from build123d import *

# Parameters (mm, degrees)
F0_W      = 36
F0_H      = 100
F1_DEPTH  = 89
F2_R      = 10.25
F3_DEPTH  = 25
F4_R      = 35.25
F5_DEPTH  = 27.5
F6_R      = 15.75
F7_DEPTH  = 3.5
F8_W      = 31.5
F8_H      = 105
F9_DEPTH  = 3.5
F10_R     = 8
F11_DEPTH = 8
F13_D     = 6.7564
F13_DEPTH = 26
F13_TIP   = 2.0298273432
F15_D     = 6.7564
F15_DEPTH = 26
F15_TIP   = 2.0298273432


with BuildPart() as f1:
    # F0 (on Top) → F1 (new body)
    with BuildSketch(Plane.XY):
        Rectangle(F0_W, F0_H)
    extrude(amount=F1_DEPTH)

    # F2 (on Front) → F3 (cut, symmetric)
    with BuildSketch(Plane.XZ):
        Circle(F2_R)
    extrude(amount=F3_DEPTH, both=True, mode=Mode.SUBTRACT)

    # F4 (on Right) → F5 (cut, symmetric)
    with BuildSketch(Plane.YZ):
        Circle(F4_R)
    extrude(amount=F5_DEPTH, both=True, mode=Mode.SUBTRACT)

    # F6 (on face) → F7 (join)
    with BuildSketch(Plane.XY.offset(89)):
        with Locations((0, 52.5)):
            Circle(F6_R)
        with Locations((0, -52.5)):
            Circle(F6_R)
    extrude(amount=-F7_DEPTH)

    # F8 (on face) → F9 (join)
    with BuildSketch(Plane.XY.offset(89)):
        Rectangle(F8_W, F8_H)
    extrude(amount=-F9_DEPTH)

    # F10 (on face) → F11 (join)
    with BuildSketch(Plane.XY.offset(89)):
        with Locations((0, 51.5)):
            Circle(F10_R)
        with Locations((0, -51.5)):
            Circle(F10_R)
    extrude(amount=-F11_DEPTH)

    # F13
    with Locations(Plane(origin=(0, 0, 0), x_dir=(1, 0, 0), z_dir=(0, 0, -1))):
        with Locations((0, 42.625)):
            Hole(F13_D / 2, depth=F13_DEPTH)
            with Locations((0, 0, -(F13_DEPTH + F13_TIP / 2))):  # 118° drill point
                Cone(0, F13_D / 2, F13_TIP, mode=Mode.SUBTRACT)

    # F15
    with Locations(Plane(origin=(0, 0, 0), x_dir=(1, 0, 0), z_dir=(0, 0, -1))):
        with Locations((0, -42.625)):
            Hole(F15_D / 2, depth=F15_DEPTH)
            with Locations((0, 0, -(F15_DEPTH + F15_TIP / 2))):  # 118° drill point
                Cone(0, F15_D / 2, F15_TIP, mode=Mode.SUBTRACT)


solid = f1.part
Can you work these out from the model? Positions are in its coordinate system, mm. A direction names the side the tool comes from. Round coordinates to 2 decimals unless told otherwise and drop trailing zeros. Loops run counter-clockwise (first coordinate to the right, second up) from the corner with the lowest first, then second, coordinate; pieces in that order, holes last. Notation, with made-up numbers: (37.25, 78.25) - (83.25, 78.25) arc R29 ccw to (83.25, 103.25) - close; hole circle Ø11 at (65.25, 27.25). An arc over 180 degrees is marked (long way). Use CSV: the item, a comma, the result in double quotes. Start each with the question number.
1) For faces 4 (the flat face through (0, 54, 81)), 5 (the flat face through (0, 61, 85.5)), 6 (the cylindrical face through (-1.6, 45.6, 13.2)), which set-ups out of +Z, -Z, +X, -X, +Y, -Y let a thin tool reach every point of the face, with its end or its side?
2) For pin 1 Ø5 at (x, y) = (1, 54) entering from -Z; pin 2 Ø1.2 at (y, z) = (51.5, 88) entering from +X; pin 3 Ø5.5 at (x, y) = (0, -42.625) entering from -Z, each with a flat end and sliding along its axis, tell me the tip position at first contact or that it passes through.
3) If we section it at D-D on x = -6: Write out the boundary of the cut face in (y, z).
4) We'd pull the mould along Y, two halves only. Please class faces 1 (the cylindrical face through (-0.346, -68.246, 87.274)), 2 (the conical face through (-0.127, -42.052, 27.677)), 3 (the flat face through (0, -39, 0)): released by +Y, released by -Y, zero draft, split by the parting line, or undercut.
5) Please list where these lines run through material, in increasing order: probe 1 along Y at (x, z) = (0, 5.5); probe 2 along Y at (x, z) = (0, 18); probe 3 along Z at (x, y) = (11, -56.5). Write a range as [from, to].
6) If we section it at B-B on y = 0: Write out the boundary of the cut face in (x, z).
7) If we section it at C-C on z = 83.5: Write out the boundary of the cut face in (x, y), plus the area to 3 significant figures.
8) If we section it at A-A on z = 22: Write out the boundary of the cut face in (x, y) (3 decimals), plus the area to 3 significant figures.
Geometry results:
1,face 4,"-Z, +X, -X, +Y"
1,face 5,"-Z, +Y"
1,face 6,"-Z"
2,pin 1,"stops at z = 81"
2,pin 2,"stops at x = 15.75"
2,pin 3,"stops at z = 26.38"
3,outline,"(-67.06, 85.5) - (-56.79, 85.5) - (-56.79, 81) - (-50, 81) - (-50, 0) - (-35.25, 0) arc R35.25 cw to (35.25, 0) - (50, 0) - (50, 81) - (56.79, 81) - (56.79, 85.5) - (67.06, 85.5) - (67.06, 89) - (-67.06, 89) - close"
4,face 1,"released by -Y"
4,face 2,"undercut"
4,face 3,"zero draft"
5,probe 1,"y = [-50, -46], [-39.25, -34.82], [34.82, 39.25], [46, 50]"
5,probe 2,"y = [-50, -46], [-39.25, -30.31], [30.31, 39.25], [46, 50]"
5,probe 3,"z = [85.5, 89]"
6,outline,"(-18, 35.25) - (18, 35.25) - (18, 89) - (-18, 89) - close"
7,outline,"(-18, -50) - (-7.86, -50) arc R8 ccw (long way) to (7.86, -50) - (18, -50) - (18, 50) - (7.86, 50) arc R8 ccw (long way) to (-7.86, 50) - (-18, 50) - close"
7,area,"3,850 mm2"
8,outline,"(-18, -50) - (18, -50) - (18, -27.542) - (-18, -27.542) - close; (-18, 27.542) - (18, 27.542) - (18, 50) - (-18, 50) - close; hole circle Ø6.756 at (0, -42.625); hole circle Ø6.756 at (0, 42.625)"
8,area,"1,550 mm2"
